Part model, mm, in its own coordinate system. Face numbers are marked on the shaded views. A direction names the side the tool comes from. Give positions to 0.01 mm unless a question says otherwise; leave off trailing zeros. Loops run counter-clockwise (first coordinate to the right, second up) from the corner with the lowest first, then second, coordinate; pieces in that order, holes last. Notation, with made-up numbers: (21, -20) -> (60, -20) arc R31 cw to (60, 7) -> close; hole circle Ø1 at (26, 42). An arc over 180 degrees is marked (long way). One line per question, with ' | ' between items.
```python
from build123d import *

# Parameters (mm, degrees)
ESQUISSE1_W             = 40
ESQUISSE1_H             = 18
BOSS_EXTRU_1_DEPTH      = 3
ESQUISSE2_W             = 3
ESQUISSE2_H             = 18
BOSS_EXTRU_2_DEPTH      = 37
ESQUISSE3_R             = 1.5
ENL_V_MAT_EXTRU_1_DEPTH = 58.384666942
ESQUISSE4_R             = 2
ENL_V_MAT_EXTRU_2_DEPTH = 58.384666942
ENL_V_MAT_EXTRU_3_DEPTH = 1.5


with BuildPart() as part:
    # Esquisse1 → Boss.-Extru.1 (new body)
    with BuildSketch(Plane.XY):
        with Locations((20, 9)):
            Rectangle(ESQUISSE1_W, ESQUISSE1_H)
    extrude(amount=BOSS_EXTRU_1_DEPTH)

    # Esquisse2 → Boss.-Extru.2 (add)
    with BuildSketch(Plane.XY.offset(3)):
        with Locations((1.5, 9)):
            Rectangle(ESQUISSE2_W, ESQUISSE2_H)
    extrude(amount=BOSS_EXTRU_2_DEPTH)

    # Esquisse3 → Enlèv. mat.-Extru.1 (cut, through all)
    with BuildSketch(Plane.XY.offset(3)):
        with Locations((14.5, 16)):
            Circle(ESQUISSE3_R)
        with Locations((29.5, 16)):
            Circle(ESQUISSE3_R)
        with Locations((14.5, 6)):
            Circle(ESQUISSE3_R)
        with Locations((29.5, 6)):
            Circle(ESQUISSE3_R)
    extrude(amount=-ENL_V_MAT_EXTRU_1_DEPTH, mode=Mode.SUBTRACT)

    # Esquisse4 → Enlèv. mat.-Extru.2 (cut, through all)
    with BuildSketch(Plane(origin=(3, 0, 0), x_dir=(0, 0, -1), z_dir=(1, 0, 0))):
        with Locations(Location((-28, 8, 0), (0, 0, 90))):
            Circle(ESQUISSE4_R)
        with Locations(Location((-13, 8, 0), (0, 0, 90))):
            Circle(ESQUISSE4_R)
    extrude(amount=-ENL_V_MAT_EXTRU_2_DEPTH, mode=Mode.SUBTRACT)

    # Esquisse5 → Enlèv. mat.-Extru.3 (cut)
    with BuildSketch(Plane.XY.offset(3)):
        Polygon((16.145448267, 8.85), (12.854551733, 8.85), (11.209103466, 6), (12.854551733, 3.15), (16.145448267, 3.15), (17.790896534, 6), align=None)
        Polygon((31.145448267, 8.85), (27.854551733, 8.85), (26.209103466, 6), (27.854551733, 3.15), (31.145448267, 3.15), (32.790896534, 6), align=None)
    extrude(amount=-ENL_V_MAT_EXTRU_3_DEPTH, mode=Mode.SUBTRACT)


solid = part.part
```
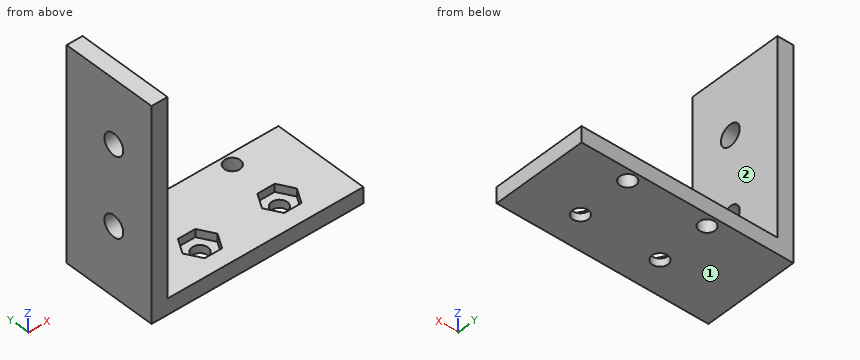
1) Drill centre lines: line 1 (Y direction, x = 14.5, z = 1.4); line 2 (Z direction, x = 24, y = 9.5). Where is each one in solid material? Low to high.
Found:
line 1: 0 to 4.5, 7.5 to 14.5, 17.5 to 18 | line 2: 0 to 3
2) Pin check, flat tips, straight feed: P1, Ø6.5, axis at x = 15, y = 5.5, coming from the +Z side; P2, Ø2.5, axis at x = 29.5, y = 6, coming from the +Z side; P3, Ø9, axis at y = 12, z = 24.5, coming from the +X side. Stop position of each tip, or through.
Found:
P1: z = 3 | P2: through | P3: x = 3
3) Saw through at B-B (y = 16). Give the cut face in (x, z).
Found:
outline: (0, 0) -> (13, 0) -> (13, 3) -> (3, 3) -> (3, 40) -> (0, 40) -> close; (16, 0) -> (28, 0) -> (28, 3) -> (16, 3) -> close; (31, 0) -> (40, 0) -> (40, 3) -> (31, 3) -> close
4) Saw through at D-D (y = 13.75). Give the cut face in (x, z), and give its area (3 significant figures).
Found:
outline: (0, 0) -> (40, 0) -> (40, 3) -> (3, 3) -> (3, 40) -> (0, 40) -> close | area: 231 mm2
5) Saw through at A-A (z = 13). Give the cut face in (x, y), and give its area (3 significant figures).
Found:
outline: (0, 0) -> (3, 0) -> (3, 6) -> (0, 6) -> close; (0, 10) -> (3, 10) -> (3, 18) -> (0, 18) -> close | area: 42.0 mm2
6) Tool access for the marked faces 1 and 2: list every direction of +Z, -Z, +X, -X, +Y, -Y with a clear straight run to the whole face (end or side of a thin tool).
Found:
face 1: -Z, +X, -X, +Y, -Y | face 2: +Z, +X, +Y, -Y
7) Saw through at C-C (x = 14.5). Give the cut face in (y, z).
Found:
outline: (0, 0) -> (4.5, 0) -> (4.5, 1.5) -> (3.15, 1.5) -> (3.15, 3) -> (0, 3) -> close; (7.5, 0) -> (14.5, 0) -> (14.5, 3) -> (8.85, 3) -> (8.85, 1.5) -> (7.5, 1.5) -> close; (17.5, 0) -> (18, 0) -> (18, 3) -> (17.5, 3) -> close
